For this review, use the dimensioned drawing (mm, ordinates from the lowest corner) and the shaded views. A direction names the side the tool comes from. Coordinates: 2 decimals unless noted, no trailing zeros. Loops run counter-clockwise (first coordinate to the right, second up) from the corner with the lowest first, then second, coordinate; pieces in that order, holes last. Notation, with made-up numbers: M -32.75,-29 L -18.75,-29 A26 cw -18.75,-13 Z; hole C 27.25,13 d3. An arc over 180 degrees is marked long. One line per item, written item: value.
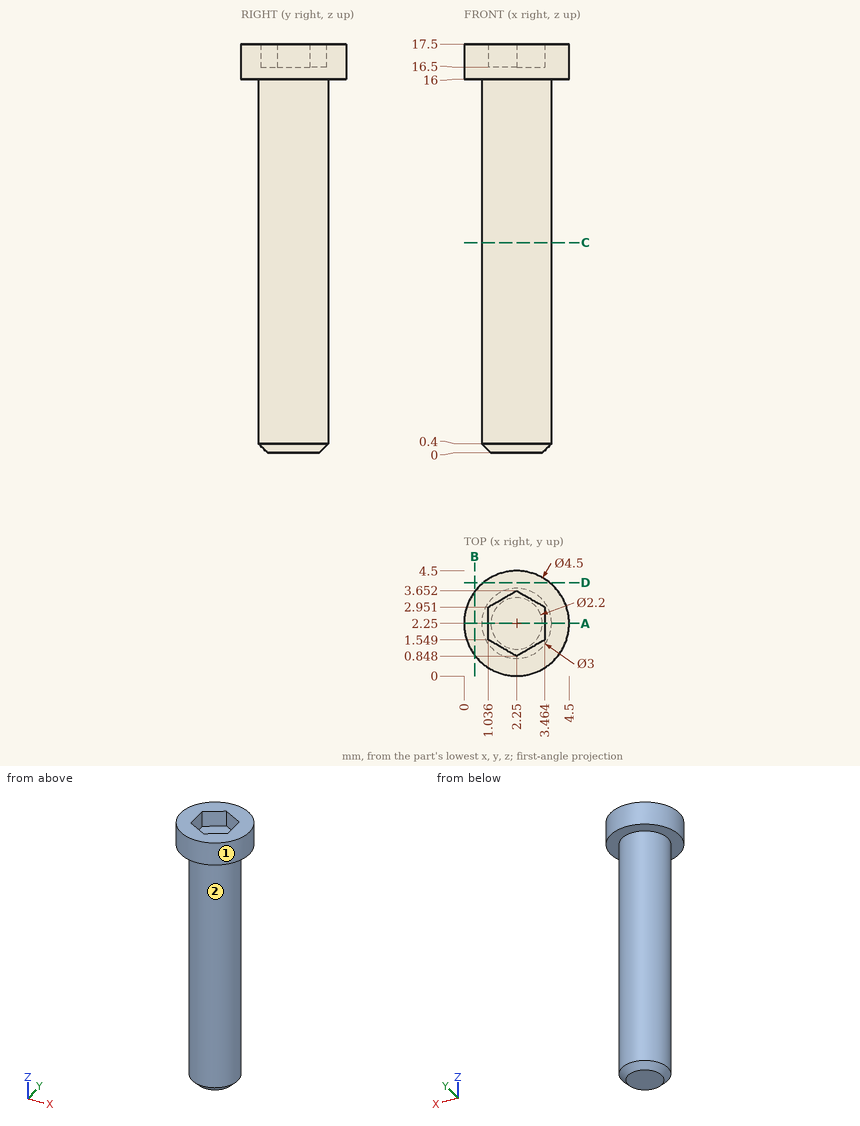
(1) Insertion check: pin 1 Ø2 at (x, z) = (2.5, 10.5) entering from -Y; pin 2 Ø1 at (y, z) = (3, 4) entering from -X. Each pin has a flat end and moves straight along its axis. Give the tip position at first contact, or say it passes through.
Checks:
pin 1: y = 0.75
pin 2: x = 0.77
(2) To check wall thickness, follow L1, parallel to Z at x = 3.35, y = 0.75; L2, parallel to Z at x = 2.6, y = 2.95; L3, parallel to Y at x = 2.2, z = 10.75. State the ranges of each line that lie inside material, in increasing order. Write a range as [from, to].
Checks:
L1: [16, 17.5]
L2: [0, 16.5]
L3: [0.75, 3.75]
(3) Add section A-A on y = 2.25. State the section outline as (x, z) points, then the cut area to 3 significant figures.
Checks:
outline: M 0,16 L 0.75,16 L 0.75,0.4 L 1.15,0 L 3.35,0 L 3.75,0.4 L 3.75,16 L 4.5,16 L 4.5,17.5 L 3.46,17.5 L 3.46,16.5 L 1.04,16.5 L 1.04,17.5 L 0,17.5 Z
area: 52.2 mm^2
(4) Add section C-C on z = 9. State the section outline as (x, y) points, then the cut area to 3 significant figures.
Checks:
outline: C 2.25,2.25 d3
area: 7.07 mm^2
(5) Add section B-B on x = 0.45. State the section outline as (y, z) points.
Checks:
outline: M 0.9,16 L 3.6,16 L 3.6,17.5 L 0.9,17.5 Z
(6) Add section D-D on y = 4. State the section outline as (x, z) points, then the cut area to 3 significant figures.
Checks:
outline: M 0.84,16 L 3.66,16 L 3.66,17.5 L 0.84,17.5 Z
area: 4.24 mm^2
(7) Tool access review of the marked faces 1 and 2: name each direction out of +Z, -Z, +X, -X, +Y, -Y from which nothing blocks a thin tool from reaching the whole face with its end or side.
Checks:
face 1: +Z, -Z
face 2: -Z
